Source: CAD feature listing. Evaluate the final solid. Frame: model axes, mm. A direction names the side the tool comes from. Round coordinates to 2 decimals unless told otherwise and drop trailing zeros. Order: outer loops, then holes, each group sorted by start corner. A loop starts at its lowest first (then second) coordinate and runs counter-clockwise, first axis right, second up. Notation, with made-up numbers: M 1,-25.75 L 48,-25.75 A14 ccw 48,-6.75 Z; hole C -6,22.25 d11. An arc over 180 degrees is marked long. Use one line per item in the form item = value. Start each with the question number.
Q1. Reachability of faces 1 (the flat face through (-27.424, -15.886, 24.65)), 2 (the flat face through (-1, -4, 50)), 3 (the flat face through (0, -3, 15)) from +Z, -Z, +X, -X, +Y, -Y: full face, straight path, thin tool, end or side. Return the list, or none.
Q2. Contact query for flat-ended pins moving along their axis: pin 1 (4 mm diameter, centred on x = 12, z = 35, fed in from -Y); pin 2 (1.8 mm diameter, centred on x = -15, z = 35, fed in from +Y); pin 3 (5 mm diameter, centred on y = -20, z = 15, fed in from +X); pin 4 (6.5 mm diameter, centred on y = -2, z = 5, fed in from +X). Output: stop coordinate, or through.
Q3. Section B-B (z = 35). Return the cut outline in (x, y), plus the area to 3 significant figures.
Q4. Section C-C (z = 9.5). Return the cut outline in (x, y), plus the area to 3 significant figures.
Q5. Section A-A (x = -15). Return the cut outline in (y, z), plus the area to 3 significant figures.
Q6. Pull-direction query (X, two-part tool) for faces 4 (the cylindrical face through (52.746, -13.03, 24.65)), 5 (the flat face through (-30, -10, 0)), 6 (the flat face through (7.5, -3, 7)); classes: pulls with the +X half, pulls with the -X half, needs draft (parallel to the pull), parting line crosses it, or undercut.
Q7. Section D-D (x = 43). Return the cut outline in (y, z), plus the area to 3 significant figures.
Q8. Material intervals for probe 1 along Z at (x, y) = (15, -4); probe 2 along X at (y, z) = (-3.75, 14); probe 3 along X at (y, z) = (-6.5, 21.5), sorted ascending.
from build123d import *

# Parameters (mm, degrees)
ESBO_O1_R                = 7.75
RESSALTO_EXTRUS_O1_DEPTH = 50
ESBO_O2_R                = 1.5
ESBO_O2_W                = 15
ESBO_O2_H                = 15
CORTE_EXTRUS_O1_DEPTH    = 30


with BuildPart() as part:
    # Esboço1 → Ressalto-extrusão1 (new body)
    with BuildSketch(Plane.XY):
        with BuildLine():
            Line((40, 0), (-40, 0))
            ThreePointArc((-40, 0), (-52.749521473, -12.749521473), (-40, -25.499042945))
            Line((-40, -25.499042945), (-30, -25.499042945))
            Line((-30, -25.499042945), (-24.77524719, -6))
            Line((-24.77524719, -6), (24.77524719, -6))
            Line((24.77524719, -6), (30, -25.499042945))
            Line((30, -25.499042945), (40, -25.499042945))
            ThreePointArc((40, -25.499042945), (52.749521473, -12.749521473), (40, 0))
        make_face()
        with Locations(Location((-40, -12.749521473, 0), (0, 0, 180))):
            Circle(ESBO_O1_R, mode=Mode.SUBTRACT)
        with Locations((40, -12.749521473)):
            Circle(ESBO_O1_R, mode=Mode.SUBTRACT)
    extrude(amount=RESSALTO_EXTRUS_O1_DEPTH)

    # Esboço2 → Corte-extrusão1 (cut)
    with BuildSketch(Plane.XZ.offset(25.499042945)):
        with Locations((15, 35)):
            Circle(ESBO_O2_R)
        with Locations((15, 15)):
            Circle(ESBO_O2_R)
        with Locations((-15, 15)):
            Circle(ESBO_O2_R)
        with Locations((-15, 35)):
            Circle(ESBO_O2_R)
        with Locations((0, 7.5)):
            Rectangle(ESBO_O2_W, ESBO_O2_H)
    extrude(amount=-CORTE_EXTRUS_O1_DEPTH, mode=Mode.SUBTRACT)


solid = part.part
Results list:
q1.face_1 = +Z, -Z, -Y
q1.face_2 = +Z, +X, -X, +Y, -Y
q1.face_3 = -Z, +Y, -Y
q2.pin_1 = -6
q2.pin_2 = through
q2.pin_3 = 51.83
q2.pin_4 = 50.31
q3.outline = M -40,-25.5 L -30,-25.5 L -24.78,-6 L -16.5,-6 L -16.5,0 L -40,0 A12.75 ccw Z; M -13.5,-6 L 13.5,-6 L 13.5,0 L -13.5,0 Z; M 16.5,-6 L 24.78,-6 L 30,-25.5 L 40,-25.5 A12.75 ccw 40,0 L 16.5,0 Z; hole C -40,-12.75 d15.5; hole C 40,-12.75 d15.5
q3.area = 1,070 mm2
q4.outline = M -40,-25.5 L -30,-25.5 L -24.78,-6 L -7.5,-6 L -7.5,0 L -40,0 A12.75 ccw Z; M 7.5,-6 L 24.78,-6 L 30,-25.5 L 40,-25.5 A12.75 ccw 40,0 L 7.5,0 Z; hole C -40,-12.75 d15.5; hole C 40,-12.75 d15.5
q4.area = 1,020 mm2
q5.outline = M -6,0 L 0,0 L 0,13.5 L -6,13.5 Z; M -6,16.5 L 0,16.5 L 0,33.5 L -6,33.5 Z; M -6,36.5 L 0,36.5 L 0,50 L -6,50 Z
q5.area = 264 mm2
q6.face_4 = pulls with the +X half
q6.face_5 = needs draft
q6.face_6 = undercut
q7.outline = M -25.14,0 L -19.9,0 L -19.9,50 L -25.14,50 Z; M -5.6,0 L -0.36,0 L -0.36,50 L -5.6,50 Z
q7.area = 525 mm2
q8.probe_1 = 0 to 13.5, 16.5 to 33.5, 36.5 to 50
q8.probe_2 = -49.03 to -16.12, -13.88 to -7.5, 7.5 to 13.88, 16.12 to 49.03
q8.probe_3 = -51.11 to -44.58, -35.42 to -24.91, 24.91 to 35.42, 44.58 to 51.11
